Input: part model. Units: mm. Frame: model coordinates. A direction names the side the tool comes from. Coordinates: 2 decimals unless noted, no trailing zeros. Write each loop counter-clockwise with the first axis right and the second up, starting at its lowest first coordinate (ties: lowest second). Pieces come first, ordered by that corner, then holes. Notation, with made-up numbers: (4, -38.5) - (57, -38.5) arc R22 ccw to (57, -16.5) - close; hole circle Ø3 at (-39.5, 9). An arc over 180 degrees is marked (long way). Put each result on its own line as item: value. Start each with the question number.
1. Pull-direction query (X, two-part tool) for faces 4 (the flat face through (0, -28, 10)), 5 (the cylindrical face through (33.713, -17.535, 4.944)), 6 (the cylindrical face through (13.716, 3.046, 27.098)); classes: released by +X, released by -X, zero draft, split by the parting line, or undercut.
2. Line query: line 1 (Y direction, x = 0, z = 25.5); line 2 (X direction, y = 0, z = 11) (3 decimals); line 3 (X direction, y = 0, z = 7.5) (3 decimals). Output: solid intervals per line, ascending.
3. Cut plane C-C, the plane z = 3. Return loops of the section in (x, y) (3 decimals).
4. Pin query (flat end, axial travel): pin 1 (2 mm diameter, centred on x = -29, y = 5.5, fed in from +Z); pin 2 (6 mm diameter, centred on y = -28, z = 3.5, fed in from -X); pin 3 (5 mm diameter, centred on y = 16, z = 6.5, fed in from +X). Return the tip coordinate at first contact, or that it passes through.
5. Cut plane D-D, the plane z = 27. Return loops of the section in (x, y).
6. Access query for faces 1 (the cylindrical face through (-5.144, -16.334, 9.074)), 2 (the flat face through (11, 11, 35)), 3 (the cylindrical face through (-17.84, 19.46, 22.34)). Directions: +Z, -Z, +X, -X, +Y, -Y. A direction counts if a zero-diameter tool reaches every point of the face in a straight line with its end or side. Return the directions, or none.
7. Cut plane A-A, the plane x = 0. Return loops of the section in (y, z) (3 decimals), and give its area (3 significant figures).
from build123d import *

# Parameters (mm, degrees)
F2_SIZE = 1
F3_R    = 1


with BuildPart() as f1:
    # F0 (on Right) → F1 (revolve)
    with BuildSketch(Plane.YZ):
        Polygon((-38, 10), (-38, 0), (-17.125, 0), (-17.125, 16.925), (-14.05, 20), (-14.05, 35), (-26.4, 35), (-26.4, 10), align=None)
    revolve(axis=Axis((0, 0, 24.570201), (0, 0, -1)))

    # F2
    f2_edges = [f1.edges().sort_by_distance(p)[0] for p in [
        (0, 38, 0),
        (0, 17.125, 0),
    ]]
    chamfer(f2_edges, length=F2_SIZE)

    # F3
    f3_edges = [f1.edges().sort_by_distance(p)[0] for p in [
        (0, 14.05, 35),
        (0, 26.4, 35),
        (0, 38, 10),
        (0, 26.4, 10),
    ]]
    fillet(f3_edges, radius=F3_R)


solid = f1.part
Report:
1. face 4: zero draft
1. face 5: split by the parting line
1. face 6: undercut
2. line 1: y = -26.4 to -14.05, 14.05 to 26.4
2. line 2: x = -26.4 to -17.125, 17.125 to 26.4
2. line 3: x = -38 to -17.125, 17.125 to 38
3. outline: circle Ø76 at (0, 0); hole circle Ø34.25 at (0, 0)
4. pin 1: stops at z = 10
4. pin 2: stops at x = -28.62
4. pin 3: stops at x = 35.52
5. outline: circle Ø52.8 at (0, 0); hole circle Ø28.1 at (0, 0)
6. face 1: -Z
6. face 2: +Z, +X, -X, +Y, -Y
6. face 3: +Z
7. outline: (-38, 1) - (-37, 0) - (-18.125, 0) - (-17.125, 1) - (-17.125, 16.925) - (-14.05, 20) - (-14.05, 34) arc R1 ccw to (-15.05, 35) - (-25.4, 35) arc R1 ccw to (-26.4, 34) - (-26.4, 11) arc R1 cw to (-27.4, 10) - (-37, 10) arc R1 ccw to (-38, 9) - close; (14.05, 20) - (17.125, 16.925) - (17.125, 1) - (18.125, 0) - (37, 0) - (38, 1) - (38, 9) arc R1 ccw to (37, 10) - (27.4, 10) arc R1 cw to (26.4, 11) - (26.4, 34) arc R1 ccw to (25.4, 35) - (15.05, 35) arc R1 ccw to (14.05, 34) - close
7. area: 980 mm^2
